from build123d import *

# Parameters (mm, degrees)
BOSS_EXTRUDE1_DEPTH         = 6.58622
M2_5_CLEARANCE_HOLE1_D      = 2.7051
M2_5_CLEARANCE_HOLE2_REACH  = 13.267
M2_5_CLEARANCE_HOLE2_BORE_R = 1.35255


with BuildPart() as part:
    # Sketch1 → Boss-Extrude1 (new body)
    with BuildSketch(Plane.XZ):
        with BuildLine():
            Line((3.04038, 0), (3.04038, 5.58038))
            Line((3.04038, 5.58038), (-3.04038, 5.58038))
            Line((-3.04038, 5.58038), (-3.04038, 0))
            ThreePointArc((-3.04038, 0), (0, -3.04038), (3.04038, 0))
        make_face()
    extrude(amount=-BOSS_EXTRUDE1_DEPTH)

    # M2.5 Clearance Hole1 (through all)
    with Locations(Plane(origin=(0, 0, 0), x_dir=(-1, 0, 0), z_dir=(0, -1, 0))):
        with Locations((0, 0)):
            Hole(M2_5_CLEARANCE_HOLE1_D / 2)

    # M2.5 Clearance Hole2 bore → M2.5 Clearance Hole2 (cut, up to next)
    with BuildSketch(Plane.XY.offset(5.58038), mode=Mode.PRIVATE) as m2_5_clearance_hole2_sk1:
        with Locations((0, 3.29311)):
            Circle(M2_5_CLEARANCE_HOLE2_BORE_R)
    m2_5_clearance_hole2_tool1 = extrude(m2_5_clearance_hole2_sk1.sketch, amount=-M2_5_CLEARANCE_HOLE2_REACH, mode=Mode.PRIVATE) & part.part
    add(m2_5_clearance_hole2_tool1.solids().sort_by_distance((0, 3.29311, 5.58038))[0], mode=Mode.SUBTRACT)


solid = part.part
Geometry: final body of the model. Coordinates: model frame, mm. Give positions to 0.01 mm unless a question says otherwise; leave off trailing zeros. Write each loop counter-clockwise with the first axis right and the second up, starting at its lowest first coordinate (ties: lowest second). Pieces come first, ordered by that corner, then holes. Notation, with made-up numbers: (-13, 75) - (42, 75) arc R32 cw to (42, 102) - close; hole circle Ø6 at (-26, -15.5). An arc over 180 degrees is marked (long way). Return JSON: item names as keys, results as strings. Group by question number.
1) First-contact query: P1, Ø1.6, axis at x = 0, z = 0, coming from the -Y side; P2, Ø3, axis at x = 2, y = 3, coming from the -Z side. Flat tips, straight axial feed; report the tip coordinate or a pass-through.
2) Section B-B on z = 0.75. Return the cut outline in (x, y).
3) Mould query, pull axis Y, two halves, no side actions, for faces 1 (the cylindrical face through (-1.35, 3.35, 3.45)), 2 (the flat face through (-3.04, 3, 3)), 3 (the flat face through (0, 0, 2)). Classes: released by +Y, released by -Y, zero draft, split by the parting line, or undercut.
4) Section A-A on x = 0. Return the cut outline in (y, z).
5) Line query: line 1 (Z direction, x = 0, y = 1.5); line 2 (Y direction, x = 0, z = 1.4); line 3 (Z direction, x = -0.25, y = 0.5). Output: solid intervals per line, ascending.
6) Section D-D on z = 4. Return the cut outline in (x, y), plus the area to 3 significant figures.
7) Section C-C on y = 4.5. Return the cut outline in (x, z), plus the area to 3 significant figures.
Filled in:
{
 "1": {"P1": "passes through", "P2": "stops at z = -3"},
 "2": {"outline": "(-3.04, 0) - (-1.13, 0) - (-1.13, 2.54) arc R1.35 cw to (-1.13, 4.04) - (-1.13, 6.59) - (-3.04, 6.59) - close; (1.13, 0) - (3.04, 0) - (3.04, 6.59) - (1.13, 6.59) - (1.13, 4.04) arc R1.35 cw to (1.13, 2.54) - close"},
 "3": {"face 1": "undercut", "face 2": "zero draft", "face 3": "released by -Y"},
 "4": {"outline": "(0, -3.04) - (6.59, -3.04) - (6.59, -1.35) - (0, -1.35) - close; (0, 1.35) - (1.94, 1.35) - (1.94, 5.58) - (0, 5.58) - close; (4.65, 1.35) - (6.59, 1.35) - (6.59, 5.58) - (4.65, 5.58) - close"},
 "5": {"line 1": "z = -3.04 to -1.35, 1.35 to 5.58", "line 2": "y = 0 to 1.94, 4.65 to 6.59", "line 3": "z = -3.03 to -1.33, 1.33 to 5.58"},
 "6": {"outline": "(-3.04, 0) - (3.04, 0) - (3.04, 6.59) - (-3.04, 6.59) - close; hole circle Ø2.71 at (0, 3.29)", "area": "34.3 mm^2"},
 "7": {"outline": "(-3.04, 0) arc R3.04 ccw to (3.04, 0) - (3.04, 5.58) - (0.61, 5.58) - (0.61, 1.21) arc R1.35 cw (long way) to (-0.61, 1.21) - (-0.61, 5.58) - (-3.04, 5.58) - close", "area": "37.5 mm^2"}
}
